The listing builds one solid part. Answer for the finished solid, in the listing's coordinates (mm). A direction names the side the tool comes from. Give positions to 0.01 mm unless a question says otherwise; leave off trailing zeros. Order: outer loops, then holes, each group sorted by start corner. A loop starts at its lowest first (then second) coordinate and runs counter-clockwise, first axis right, second up. Notation, with made-up numbers: M 33,38.5 L 44,38.5 A33 ccw 44,72.5 Z; hole C 88.5,-5 d7. An arc over 180 degrees is marked long. Answer as a JSON object with one key per item and string values. Group by question number.
```python
from build123d import *

# Parameters (mm, degrees)
AUFSATZ_LINEAR_AUSTRAGEN1_DEPTH = 3
SCHNITT_LINEAR_AUSTRAGEN1_REACH = 5


with BuildPart() as part:
    # Skizze1 → Aufsatz-Linear austragen1 (new body)
    with BuildSketch(Plane(origin=(0, 0, 0), x_dir=(1, 0, 0), z_dir=(0, 1, 0))):
        Polygon((0, 0), (8.199374, 0), (8.199374, 3.000248), (16.400272, 3.000248), (16.400272, 0), (24.599646, 0), (24.599646, 3.000248), (32.80029, 3.000248), (32.80029, 0), (37.999416, 0), (37.999416, 20), (32.80029, 20), (32.80029, 17.000006), (24.599646, 17.000006), (24.599646, 20), (16.400272, 20), (16.400272, 17.000006), (8.199374, 17.000006), (8.199374, 20), (0, 20), align=None)
    extrude(amount=AUFSATZ_LINEAR_AUSTRAGEN1_DEPTH)

    # Skizze2 → Schnitt-Linear austragen1 (cut, up to next)
    with BuildSketch(Plane.XZ, mode=Mode.PRIVATE) as schnitt_linear_austragen1_sk1:
        with BuildLine():
            Line((11.499959, -20), (11.499959, -11.5))
            ThreePointArc((11.499959, -11.5), (12.999959, -10), (14.499959, -11.5))
            Line((14.499959, -11.5), (14.499959, -20))
            Line((14.499959, -20), (11.499959, -20))
        make_face()
    schnitt_linear_austragen1_tool1 = extrude(schnitt_linear_austragen1_sk1.sketch, amount=-SCHNITT_LINEAR_AUSTRAGEN1_REACH, mode=Mode.PRIVATE) & part.part
    add(schnitt_linear_austragen1_tool1.solids().sort_by_distance((12.999959, 0, -15.155161))[0], mode=Mode.SUBTRACT)
    # Skizze2 → Schnitt-Linear austragen1 (cut, up to next)
    with BuildSketch(Plane.XZ, mode=Mode.PRIVATE) as schnitt_linear_austragen1_sk2:
        with BuildLine():
            Line((26.499959, -20), (29.499959, -20))
            Line((29.499959, -20), (29.499959, -11.5))
            ThreePointArc((29.499959, -11.5), (27.999959, -10), (26.499959, -11.5))
            Line((26.499959, -11.5), (26.499959, -20))
        make_face()
    schnitt_linear_austragen1_tool2 = extrude(schnitt_linear_austragen1_sk2.sketch, amount=-SCHNITT_LINEAR_AUSTRAGEN1_REACH, mode=Mode.PRIVATE) & part.part
    add(schnitt_linear_austragen1_tool2.solids().sort_by_distance((27.999959, 0, -15.155161))[0], mode=Mode.SUBTRACT)
    # Skizze2 → Schnitt-Linear austragen1 (cut, up to next)
    with BuildSketch(Plane.XZ, mode=Mode.PRIVATE) as schnitt_linear_austragen1_sk3:
        with BuildLine():
            Line((18.999959, -10), (21.999959, -10))
            ThreePointArc((21.999959, -10), (23.060619172, -10.439339828), (23.499959, -11.5))
            Line((23.499959, -11.5), (23.499959, -13.500006))
            ThreePointArc((23.499959, -13.500006), (23.060619172, -14.560666172), (21.999959, -15.000006))
            Line((21.999959, -15.000006), (18.999959, -15.000006))
            ThreePointArc((18.999959, -15.000006), (17.939298828, -14.560666172), (17.499959, -13.500006))
            Line((17.499959, -13.500006), (17.499959, -11.5))
            ThreePointArc((17.499959, -11.5), (17.939298828, -10.439339828), (18.999959, -10))
        make_face()
    schnitt_linear_austragen1_tool3 = extrude(schnitt_linear_austragen1_sk3.sketch, amount=-SCHNITT_LINEAR_AUSTRAGEN1_REACH, mode=Mode.PRIVATE) & part.part
    add(schnitt_linear_austragen1_tool3.solids().sort_by_distance((20.499959, 0, -12.500003))[0], mode=Mode.SUBTRACT)


solid = part.part
```
Item 1: Consider probe 1 along X at (y, z) = (2.35, -15.5); probe 2 along X at (y, z) = (1.55, -19); probe 3 along Z at (x, y) = (25, 2.05). Determine where each line is inside the solid, lowest interval first. Write a range as from..to.
Item 2: Section B-B (x = 23) is taken. Determine the outline of the cut face in (y, z), and give its area (3 significant figures).
Item 3: A flat-ended cylindrical pin translates along its axis: P1, Ø1.5, axis at x = 25.5, y = 2, coming from the -Z side. Find the tip coordinate at first contact, or state that the pin passes through.
Item 4: Section A-A (z = -1.5) is taken. Determine the outline of the cut face in (x, y).
Item 5: A tool of negligible diameter and unlimited length cuts with its end or side. For faces 5 (the flat face through (32.8, 1, -2)), 6 (the flat face through (37.999, 1, -10)), 7 (the flat face through (11.5, 1, -14)), 8 (the flat face through (35, 1, 0)), 9 (the cylindrical face through (17.95, 1.48, -14.57)), from which of +Z, -Z, +X, -X, +Y, -Y can it reach the whole face along a straight path? Write none if from no direction.
Item 6: Section C-C (z = -14.5) is taken. Determine the outline of the cut face in (x, y), and give its area (3 significant figures).
Item 7: Section D-D (x = 10) is taken. Determine the outline of the cut face in (y, z), and give its area (3 significant figures).
Item 8: Determine the mould class of faces 1 (the flat face through (21, 1, -20)), 2 (the flat face through (8.199, 1, -18)), 3 (the flat face through (17.5, 1, -13)), 4 (the flat face through (23.5, 1, -12)) for opening direction Z: released by +Z, released by -Z, zero draft, split by the parting line, or undercut.
Values found:
{
 "1": {"probe 1": "x = 0..11.5, 14.5..26.5, 29.5..38", "probe 2": "x = 0..8.2, 16.4..24.6, 32.8..38", "probe 3": "z = -17..-3"},
 "2": {"outline": "M 0,-20 L 3,-20 L 3,-14.62 L 0,-14.62 Z; M 0,-10.38 L 3,-10.38 L 3,0 L 0,0 Z", "area": "47.3 mm^2"},
 "3": {"P1": "stops at z = -17"},
 "4": {"outline": "M 0,0 L 8.2,0 L 8.2,3 L 0,3 Z; M 16.4,0 L 24.6,0 L 24.6,3 L 16.4,3 Z; M 32.8,0 L 38,0 L 38,3 L 32.8,3 Z"},
 "5": {"face 5": "+Z, +Y, -Y", "face 6": "+Z, -Z, +X, +Y, -Y", "face 7": "-Z, +Y, -Y", "face 8": "+Z, +X, -X, +Y, -Y", "face 9": "+Y, -Y"},
 "6": {"outline": "M 0,0 L 11.5,0 L 11.5,3 L 0,3 Z; M 14.5,0 L 17.88,0 L 17.88,3 L 14.5,3 Z; M 23.12,0 L 26.5,0 L 26.5,3 L 23.12,3 Z; M 29.5,0 L 38,0 L 38,3 L 29.5,3 Z", "area": "80.3 mm^2"},
 "7": {"outline": "M 0,-17 L 3,-17 L 3,-3 L 0,-3 Z", "area": "42.0 mm^2"},
 "8": {"face 1": "released by -Z", "face 2": "zero draft", "face 3": "undercut", "face 4": "undercut"}
}
